Solid Edge part; units mm, degrees
sketch "Sketch1" plane through (0, 0, 0) normal (0, 0, 1) x (1, 0, 0)
  circle A0 centre (0, 0) radius 28
  circle A1 centre (0, 0) radius 4.075
extrude "Protrusion1" add sketch "Sketch1" along normal blind 5
sketch "Sketch2" plane through (0, 0, 5) normal (0, 0, 1) x (1, 0, 0)
  circle A0 centre (-23, 0) radius 4.125
extrude "ExtrudedCutout_1" cut sketch "Sketch2" against normal blind 3
sketch "Sketch3" plane through (0, 0, 5) normal (0, 0, 1) x (1, 0, 0)
  circle A0 centre (-23, 0) radius 5
  circle A1 centre (-23, 0) radius 4.125
extrude "ExtrudedProtrusion_2" add sketch "Sketch3" along normal blind 1.5
sketch "Sketch4" plane through (0, 0, 5) normal (0, 0, 1) x (1, 0, 0)
  circle A0 centre (0, 0) radius 4.075
  circle A1 centre (0, 0) radius 11
extrude "ExtrudedProtrusion_3" add sketch "Sketch4" along normal blind 17
pattern_circular "Pattern1" count 5 over 360 about axis through (0, 0, 0) along (0, 0, -1) of "ExtrudedCutout_1", "ExtrudedProtrusion_2"
sketch "Sketch5" plane through (0, 0, 22) normal (0, 0, 1) x (1, 0, 0)
  circle A0 centre (-8, 0) radius 1.625
  circle A1 centre (0, 8) radius 1.625
  circle A2 centre (8, 0) radius 1.625
  circle A3 centre (0, -8) radius 1.625
extrude "Cutout1" cut sketch "Sketch5" against normal up to next
sketch "Sketch6" plane through (0, 0, 0) normal (0, 0, -1) x (1, 0, 0)
  circle A0 centre (8, 0) radius 2.25
  circle A1 centre (8, 0) radius 1.625
  circle A2 centre (0, -8) radius 2.25
  circle A3 centre (0, -8) radius 1.625
  circle A4 centre (0, 8) radius 2.25
  circle A5 centre (0, 8) radius 1.625
  circle A6 centre (-8, 0) radius 2.25
  circle A7 centre (-8, 0) radius 1.625
extrude "Cutout2" cut sketch "Sketch6" against normal blind 5.25
chamfer "Chamfer_3" distance 0.8 distance2 0.4 4 edges at (-2.25, -8, 5.25) (5.75, 0, 5.25) (-2.25, 8, 5.25) (-10.25, 0, 5.25) measured on face at (1.545, -9.455, 5.25) measured on face at (-6.455, -1.455, 5.25) measured on face at (9.545, -1.455, 5.25) measured on face at (1.545, 6.545, 5.25) measured on face at (1.545, -9.455, 5.25) measured on face at (-6.455, -1.455, 5.25) measured on face at (9.545, -1.455, 5.25) measured on face at (1.545, 6.545, 5.25) measured on face at (1.545, -9.455, 5.25) measured on face at (-6.455, -1.455, 5.25) measured on face at (9.545, -1.455, 5.25) measured on face at (1.545, 6.545, 5.25) measured on face at (1.545, -9.455, 5.25) measured on face at (-6.455, -1.455, 5.25) measured on face at (9.545, -1.455, 5.25) measured on face at (1.545, 6.545, 5.25)
sketch "Sketch7" plane through (7.7782, 7.7782, 13.5) normal (0.7071068, 0.7071068, 0) x (0, 0, -1)
  circle A0 centre (2.5, 0) radius 1.7
extrude "Cutout3" cut sketch "Sketch7" against normal up to next
sketch "Sketch8" plane through (7.7782, 7.7782, 13.5) normal (0.7071068, 0.7071068, 0) x (0, 0, -1)
  circle A0 centre (2.5, 0) radius 1.7
  circle A1 centre (2.5, 0) radius 2.275
extrude "ExtrudedProtrusion_7" cut sketch "Sketch8" against normal blind 5.25
sketch "Sketch9" plane through (-7.7782, -7.7782, 13.5) normal (-0.7071068, -0.7071068, 0) x (0, 0, -1)
  circle A0 centre (2.5, 0) radius 1.7
  circle A1 centre (2.5, 0) radius 2.275
extrude "ExtrudedCutout_12" cut sketch "Sketch9" against normal blind 5.25
sketch "Sketch10" plane through (-7.7782, -7.7782, 13.5) normal (-0.7071068, -0.7071068, 0) x (0, 0, -1)
  circle A0 centre (2.5, 0) radius 1.7
extrude "Cutout4" cut sketch "Sketch10" against normal up to next
Can you work these out from the model? Positions are in its coordinate system, mm. A direction names the side the tool comes from. Give positions to 0.01 mm unless a question says otherwise; leave off trailing zeros. Write each loop counter-clockwise with the first axis right and the second up, starting at its lowest first coordinate (ties: lowest second). Pieces come first, ordered by that corner, then holes. Notation, with made-up numbers: M 74,-4 L 104,-4 A13 ccw 104,21 Z; hole C 82,-11 d9. An arc over 180 degrees is marked long. Answer in a Markdown table with one row per item. Add a question column.
Item 1: Imagine slicing it at C-C, the plane y = -12. Write out the boundary of the cut face in (x, z), plus the area to 3 significant figures.
Item 2: On a 3-axis mill with a long thin cutter (end or side, diameter ignored), from which of +Z, -Z, +X, -X, +Y, -Y can I reach the whole of each face in a straight line? I mean faces 1 (the flat face through (-11, -20, 6.5)), 2 (the cylindrical face through (-3.81, -2.89, 9.43)), 3 (the cylindrical face through (5.752, -0.099, 2.391)), 4 (the cylindrical face through (16.453, 10.001, 4.219)). Say none if no direction works.
Item 3: Imagine slicing it at D-D, the plane x = -23.5. Write out the boundary of the cut face in (y, z), plus the area to 3 significant figures.
Item 4: For pin 1 Ø3 at (y, z) = (-20.5, 2.5) entering from -X; pin 2 Ø11 at (x, y) = (-8.5, 22.5) entering from +Z; pin 3 Ø2 at (x, z) = (-1, 9) entering from -Y, each with a flat end and sliding along its axis, tell me the tip position at first contact or that it passes through.
Item 5: Imagine slicing it at A-A, the plane x = 0. State how many separate pieces and enclosed holes the cut face has, plus the area to 3 significant figures.
Item 6: Imagine slicing it at B-B, the plane z = 17.75. Write out the boundary of the cut face in (x, y) (3 decimals), plus the area to 3 significant figures.
Item 7: We'd pull the mould along Y, two halves only. Please class faces 5 (the cylindrical face through (25.865, 10.724, 2.465)), 6 (the flat face through (0, -5, 22)), 7 (the cylindrical face through (-9.623, 0.071, 13.699)): released by +Y, released by -Y, zero draft, split by the parting line, or undercut.
Item 8: Please list where these lines run through material, in increasing order: L1, parallel to Y at x = 0, z = 5.25 (3 decimals); L2, parallel to Y at x = 0, z = 2.35 (3 decimals); L3, parallel to Z at x = -10, y = -9.
Evaluation:
| question | item | result |
|---|---|---|
| 1 | outline | M -25.3,0 L 25.3,0 L 25.3,5 L 23.37,5 L 23.37,6.5 L 22.44,6.5 L 22.44,2 L 14.77,2 L 14.77,6.5 L 13.84,6.5 L 13.84,5 L -25.3,5 Z |
| 1 | area | 233 mm² |
| 2 | face 1 | +Z, +X, -X, -Y |
| 2 | face 2 | none |
| 2 | face 3 | -Z |
| 2 | face 4 | +Z |
| 3 | outline | M -15.22,0 L 15.22,0 L 15.22,5 L 4.97,5 L 4.97,6.5 L 4.09,6.5 L 4.09,2 L -4.09,2 L -4.09,6.5 L -4.97,6.5 L -4.97,5 L -15.22,5 Z |
| 3 | area | 130 mm² |
| 4 | pin 1 | stops at x = -20.57 |
| 4 | pin 2 | stops at z = 6.5 |
| 4 | pin 3 | stops at y = -11 |
| 5 | separate pieces | 4 |
| 5 | enclosed holes | 0 |
| 5 | area | 319 mm² |
| 6 | outline | C 0,0 d22; hole C -8,0 d3.25; hole C 0,0 d8.15; hole C 0,-8 d3.25; hole C 0,8 d3.25; hole C 8,0 d3.25 |
| 6 | area | 295 mm² |
| 7 | face 5 | split by the parting line |
| 7 | face 6 | zero draft |
| 7 | face 7 | undercut |
| 8 | L1 | y = -11 to -9.625, -6.375 to -4.075, 4.075 to 6.375, 9.625 to 11 |
| 8 | L2 | y = -28 to -10.25, -5.75 to -4.075, 4.075 to 5.75, 10.25 to 28 |
| 8 | L3 | z = 0 to 5 |
